```python
from build123d import *

# Parameters (mm, degrees)
SKETCH_1_R      = 2.5
EXTRUDE_1_DEPTH = 4
FILLET_1_R      = 4


with BuildPart() as part:
    # ｽｹｯﾁ1 → ﾎﾞｽ - 押し出し1 (new body)
    with BuildSketch(Plane.XY):
        Polygon((-6.9, 14.13928001), (6.9, 14.13928001), (13.299484522, -1.7), (3.6, -7.3), (-3.6, -7.3), (-13.299484522, -1.7), align=None)
        Circle(SKETCH_1_R, mode=Mode.SUBTRACT)
        Polygon((2.541237363, 8.910793136), (6.249972781, 10.409219509), (9.808735418, 1.600972891), (6.1, 0.102546517), align=None, mode=Mode.SUBTRACT)
        Polygon((-6.1, 0.102546517), (-2.541237363, 8.910793136), (-6.249972781, 10.409219509), (-9.808735418, 1.600972891), align=None, mode=Mode.SUBTRACT)
    extrude(amount=EXTRUDE_1_DEPTH)

    # ﾌｨﾚｯﾄ1
    fillet_1_edges = [part.edges().sort_by_distance(p)[0] for p in [
        (13.299484522, -1.7, 2),
        (3.6, -7.3, 2),
        (-3.6, -7.3, 2),
        (-13.299484522, -1.7, 2),
        (-6.9, 14.13928001, 2),
        (6.9, 14.13928001, 2),
    ]]
    fillet(fillet_1_edges, radius=FILLET_1_R)


solid = part.part
```
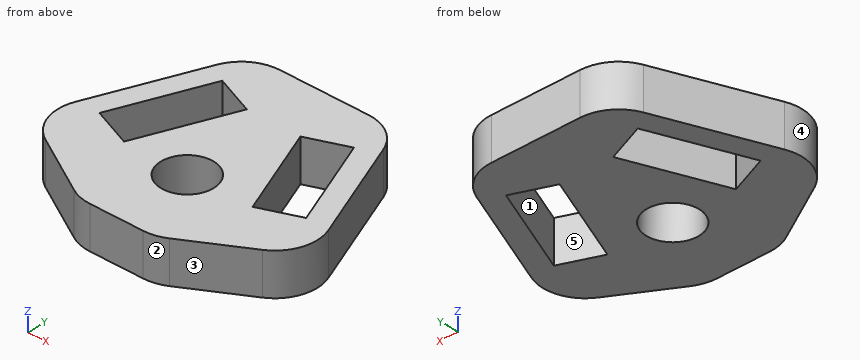
Geometry: final body of the model. Coordinates: model frame, mm. Face numbers are marked on the shaded views. A direction names the side the tool comes from. Coordinates: 2 decimals unless noted, no trailing zeros. Order: outer loops, then holes, each group sorted by start corner. A loop starts at its lowest first (then second) coordinate and runs counter-clockwise, first axis right, second up. Notation, with made-up numbers: (60, 78.5) -> (74, 78.5) arc R17 cw to (74, 91.5) -> close; hole circle Ø1 at (71.25, -21.75). An arc over 180 degrees is marked (long way). Use CSV: the item, a comma, the result in double quotes.
1) Mould query, pull axis X, two halves, no side actions, for the marked faces 3, 4 and 5. Classes: +X half, -X half, draft (parallel to the pull), parting line (faces both ways), or undercut.
Findings:
face 3,"+X half"
face 4,"-X half"
face 5,"undercut"
2) Section C-C on z = 1.45. Output: boundary loops of the cut face in (x, y).
Findings:
outline,"(-12, 1.52) arc R4 ccw to (-10.29, -3.44) -> (-4.53, -6.76) arc R4 ccw to (-2.53, -7.3) -> (2.53, -7.3) arc R4 ccw to (4.53, -6.76) -> (10.29, -3.44) arc R4 ccw to (12, 1.52) -> (7.91, 11.64) arc R4 ccw to (4.2, 14.14) -> (-4.2, 14.14) arc R4 ccw to (-7.91, 11.64) -> close; hole (-9.81, 1.6) -> (-6.1, 0.1) -> (-2.54, 8.91) -> (-6.25, 10.41) -> close; hole circle Ø5 at (0, 0); hole (2.54, 8.91) -> (6.1, 0.1) -> (9.81, 1.6) -> (6.25, 10.41) -> close"
3) Line query: line 1 (X direction, y = 2, z = 0.95); line 2 (Y direction, x = 0, z = 1.6); line 3 (X direction, y = 7.25, z = 1.7). Output: solid intervals per line, ascending.
Findings:
line 1,"x = -11.8 to -9.65, -5.33 to -1.5, 1.5 to 5.33, 9.65 to 11.8"
line 2,"y = -7.3 to -2.5, 2.5 to 14.14"
line 3,"x = -9.68 to -7.53, -3.21 to 3.21, 7.53 to 9.68"
4) Section B-B on y = 4.25. Output: boundary loops of the cut face in (x, z).
Findings:
outline,"(-10.9, 0) -> (-8.74, 0) -> (-8.74, 4) -> (-10.9, 4) -> close; (-4.42, 0) -> (4.42, 0) -> (4.42, 4) -> (-4.42, 4) -> close; (8.74, 0) -> (10.9, 0) -> (10.9, 4) -> (8.74, 4) -> close"
5) Section D-D on y = -0.5. Output: boundary loops of the cut face in (x, z).
Findings:
outline,"(-12.25, 0) -> (-2.45, 0) -> (-2.45, 4) -> (-12.25, 4) -> close; (2.45, 0) -> (12.25, 0) -> (12.25, 4) -> (2.45, 4) -> close"
6) Pin query (flat end, axial travel): pin 1 Ø2 at (x, z) = (9, 1) entering from +Y; pin 2 Ø1 at (y, z) = (-2, 1.5) entering from -X. Return the tip coordinate at first contact, or that it passes through.
Findings:
pin 1,"stops at y = 11.42"
pin 2,"stops at x = -11.99"
7) Access query for the marked faces 1 and 2. Directions: +Z, -Z, +X, -X, +Y, -Y. A direction counts if a zero-diameter tool reaches every point of the face in a straight line with its end or side. Return the directions, or none.
Findings:
face 1,"+Z, -Z"
face 2,"+Z, -Z, +X, -Y"
8) Section A-A on x = 0. Output: boundary loops of the cut face in (y, z), then the cut area to 3 significant figures.
Findings:
outline,"(-7.3, 0) -> (-2.5, 0) -> (-2.5, 4) -> (-7.3, 4) -> close; (2.5, 0) -> (14.14, 0) -> (14.14, 4) -> (2.5, 4) -> close"
area,"65.8 mm^2"
